Work out the finished part from the listing and answer in its coordinate system (mm). Round coordinates to 2 decimals unless told otherwise and drop trailing zeros. Order: outer loops, then holes, each group sorted by start corner. A loop starts at its lowest first (then second) coordinate and runs counter-clockwise, first axis right, second up. Notation, with made-up numbers: (50.25, 47) - (75.25, 47) arc R28 cw to (75.25, 68) - close; hole circle Ø3 at (-30.5, -34). An arc over 180 degrees is marked (long way). Answer in a Markdown table with one row per item.
from build123d import *

# Parameters (mm, degrees)
SKETCH1_W           = 95
SKETCH1_H           = 70
BOSS_EXTRUDE1_DEPTH = 3
SKETCH2_W           = 4
SKETCH2_H           = 10
SKETCH2_W_2         = 15
SKETCH2_H_2         = 4
BOSS_EXTRUDE2_DEPTH = 3


with BuildPart() as part:
    # Sketch1 → Boss-Extrude1 (new body)
    with BuildSketch(Plane.XY):
        with Locations((-47.5, 35)):
            Rectangle(SKETCH1_W, SKETCH1_H)
    extrude(amount=BOSS_EXTRUDE1_DEPTH)

    # Sketch2 → Boss-Extrude2 (add)
    with BuildSketch(Plane.XY.offset(3)):
        Polygon((0, 15), (4, 15), (4, 0), (4, -4), (0, -4), (-15, -4), (-15, 0), (0, 0), align=None)
        with Locations((2, 35)):
            Rectangle(SKETCH2_W, SKETCH2_H)
        Polygon((-95, 70), (-80, 70), (-80, 74), (-95, 74), (-99, 74), (-99, 70), (-99, 55), (-95, 55), align=None)
        Polygon((0, 74), (-15, 74), (-15, 70), (0, 70), (0, 55), (4, 55), (4, 70), (4, 74), align=None)
        with Locations((-57.5, 72)):
            Rectangle(SKETCH2_W_2, SKETCH2_H_2)
        with Locations((-37.5, 72)):
            Rectangle(SKETCH2_W_2, SKETCH2_H_2)
        with Locations((-37.5, -2)):
            Rectangle(SKETCH2_W_2, SKETCH2_H_2)
        with Locations((-57.5, -2)):
            Rectangle(SKETCH2_W_2, SKETCH2_H_2)
        Polygon((-80, -4), (-95, -4), (-99, -4), (-99, 0), (-99, 15), (-95, 15), (-95, 0), (-80, 0), align=None)
        with Locations((-97, 35)):
            Rectangle(SKETCH2_W, SKETCH2_H)
    extrude(amount=-BOSS_EXTRUDE2_DEPTH)


solid = part.part
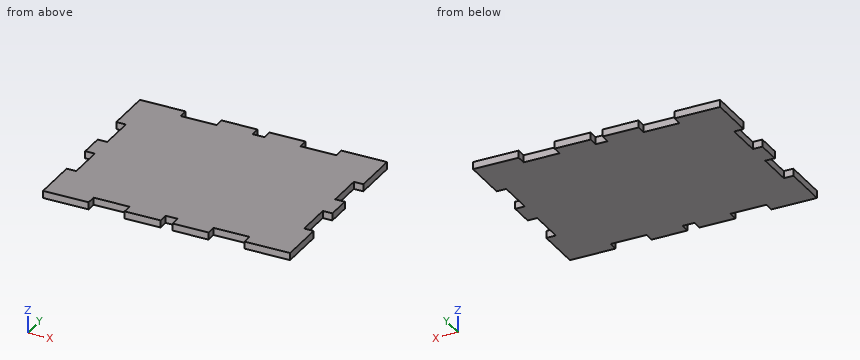
1) Find the intervals of material crossed by probe 1 along Y at (x, z) = (-67, 1.2); probe 2 along X at (y, z) = (40.5, 0.65), in increasing order. Write a range as from..to.
Filled in:
| item | result |
|---|---|
| probe 1 | y = 0..70 |
| probe 2 | x = -95..0 |
2) Each of these flat-tipped pins is pushed along its axis until it touches: pin 1 (0.9 mm diameter, centred on x = -74.5, z = 1.5, fed in from +Y); pin 2 (1.5 mm diameter, centred on x = -24, z = 2, fed in from -Y); pin 3 (1.5 mm diameter, centred on y = 46, z = 1, fed in from +X). Where does it stop, or does it pass through?
Filled in:
| item | result |
|---|---|
| pin 1 | stops at y = 70 |
| pin 2 | stops at y = 0 |
| pin 3 | stops at x = 0 |
3) Find section A-A, the plane y = 43. Give the vertices of the cut face in (x, z).
Filled in:
| item | result |
|---|---|
| outline | (-95, 0) - (0, 0) - (0, 3) - (-95, 3) - close |
4) Find section B-B, the plane x = -22. Give the vertices of the cut face in (y, z), then the cut area to 3 significant figures.
Filled in:
| item | result |
|---|---|
| outline | (0, 0) - (70, 0) - (70, 3) - (0, 3) - close |
| area | 210 mm^2 |
